Geometry: final body of the model. Coordinates: model frame, mm. Give positions to 0.01 mm unless a question says otherwise; leave off trailing zeros. Order: outer loops, then holes, each group sorted by start corner. A loop starts at its lowest first (then second) coordinate and runs counter-clockwise, first axis right, second up. Notation, with made-up numbers: (22, 75) - (55, 75) arc R11 cw to (55, 80) - close; hole circle Ø5 at (48.5, 2). An arc over 180 degrees is marked (long way). One line per item, written item: value.
```python
from build123d import *

# Parameters (mm, degrees)
SKETCH_1_W          = 40
SKETCH_1_H          = 40
EXTRUDE_1_DEPTH     = 40
CUT_EXTRUDE_1_DEPTH = 77.035731628
CUT_EXTRUDE_2_DEPTH = 62.629021291
FILLET_1_R          = 2


with BuildPart() as part:
    # Эскиз1 → Бобышка-Вытянуть1 (new body)
    with BuildSketch(Plane(origin=(0, 0, 0), x_dir=(1, 0, 0), z_dir=(0, 1, 0))):
        with Locations((-30.807799443, -4.456824513)):
            Rectangle(SKETCH_1_W, SKETCH_1_H)
    extrude(amount=EXTRUDE_1_DEPTH)

    # Эскиз2 → Вырез-Вытянуть1 (cut, through all)
    with BuildSketch(Plane(origin=(0, 0, -15.543175487), x_dir=(-1, 0, 0), z_dir=(0, 0, -1))):
        Polygon((10.807799443, 40), (10.807799443, 0), (20.807799443, 0), align=None)
    extrude(amount=-CUT_EXTRUDE_1_DEPTH, mode=Mode.SUBTRACT)

    # Эскиз3 → Вырез-Вытянуть2 (cut, through all)
    with BuildSketch(Plane.ZY.offset(50.807799443)):
        Polygon((24.456824513, 0), (14.456824513, 0), (24.456824513, 40), align=None)
    extrude(amount=-CUT_EXTRUDE_2_DEPTH, mode=Mode.SUBTRACT)

    # Скругление1
    fillet_1_edges = [part.edges().sort_by_distance(p)[0] for p in [
        (-15.807799443, 20, -15.543175487),
        (-15.807799443, 20, 19.456824513),
        (-50.807799443, 20, 19.456824513),
        (-50.807799443, 20, -15.543175487),
    ]]
    fillet(fillet_1_edges, radius=FILLET_1_R)


solid = part.part
```
1) Material intervals for line 1 along X through (y, z) = (21, 13.5); line 2 along X through (y, z) = (34, 13); line 3 along Z through (x, y) = (-34, 2), sorted ascending.
Answers below:
line 1: -50.81 to -15.56
line 2: -50.81 to -12.31
line 3: -15.54 to 14.96
2) Section B-B, the plane x = -34.5. Return loops of the section in (y, z), then the cut area to 3 significant figures.
Answers below:
outline: (0, -15.54) - (40, -15.54) - (40, 24.46) - (0, 14.46) - close
area: 1,400 mm^2
3) First-contact query: pin 1 (1 mm diameter, centred on y = 34, z = 11, fed in from +X); pin 2 (3 mm diameter, centred on y = 16, z = 1, fed in from +X). Flat tips, straight axial feed; report the tip coordinate or a pass-through.
Answers below:
pin 1: x = -12.18
pin 2: x = -16.43
4) Section A-A, the plane z = 6.5. Return loops of the section in (x, y), then the cut area to 3 significant figures.
Answers below:
outline: (-50.81, 0) - (-20.81, 0) - (-10.81, 40) - (-50.81, 40) - close
area: 1,400 mm^2
